from build123d import *

# Parameters (mm, degrees)
SKETCH_1_R       = 11
EXTRUDE_1_DEPTH  = 14
SKETCH_3_R       = 10.95
SKETCH_3_R_2     = 10.9
EXTRUDE_6_DEPTH  = 26
SKETCH_5_R       = 11
SKETCH_5_R_2     = 10.95
SKETCH_5_R_3     = 10.9
EXTRUDE_7_DEPTH  = 11
SKETCH_6_R       = 7
SKETCH_6_R_2     = 6.25
EXTRUDE_8_DEPTH  = 16.5
SKETCH_6_3_R     = 3.75
SKETCH_6_3_R_2   = 3.25
EXTRUDE_9_DEPTH  = 15
FILLET_1_R       = 0.5
FILLET_2_R       = 0.5
SKETCH_8_R       = 9
EXTRUDE_10_DEPTH = 15
SKETCH_9_R       = 4.762822891
EXTRUDE_11_DEPTH = 15
CHAMFER_1_SIZE   = 4
CHAMFER_1_SIZE2  = 2.800830153


with BuildPart() as part:
    # Sketch 1 → Extrude 1 (new body)
    with BuildSketch(Plane(origin=(0, 0, 0), x_dir=(1, 0, 0), z_dir=(0, 1, 0))):
        with Locations(Location((0, 0, 0), (0, 0, 270))):
            Circle(SKETCH_1_R)
    extrude(amount=EXTRUDE_1_DEPTH)

    # Sketch 3 → Extrude 6 (add)
    with BuildSketch(Plane(origin=(0, 14, 0), x_dir=(1, 0, 0), z_dir=(0, 1, 0))):
        with Locations(Location((0, 0, 0), (0, 0, 90))):
            Circle(SKETCH_3_R)
        with Locations(Location((0, 0, 0), (0, 0, 90))):
            Circle(SKETCH_3_R_2, mode=Mode.SUBTRACT)
    extrude(amount=EXTRUDE_6_DEPTH)

    # Sketch 5 → Extrude 7 (add)
    # profile 1 of 3: a face of its own
    with BuildSketch(Plane(origin=(0, 40, 0), x_dir=(1, 0, 0), z_dir=(0, 1, 0))):
        with Locations(Location((0, 0, 0), (0, 0, 270))):
            Circle(SKETCH_5_R)
        with Locations(Location((0, 0, 0), (0, 0, 90))):
            Circle(SKETCH_5_R_2, mode=Mode.SUBTRACT)
    # profile 2 of 3: a face of its own
    with BuildSketch(Plane(origin=(0, 40, 0), x_dir=(1, 0, 0), z_dir=(0, 1, 0))):
        with Locations(Location((0, 0, 0), (0, 0, 90))):
            Circle(SKETCH_5_R_2)
        with Locations(Location((0, 0, 0), (0, 0, 90))):
            Circle(SKETCH_5_R_3, mode=Mode.SUBTRACT)
    # profile 3 of 3: a face of its own
    with BuildSketch(Plane(origin=(0, 40, 0), x_dir=(1, 0, 0), z_dir=(0, 1, 0))):
        with Locations(Location((0, 0, 0), (0, 0, 90))):
            Circle(SKETCH_5_R_3)
    extrude(amount=EXTRUDE_7_DEPTH)

    # Sketch 6 → Extrude 8 (add)
    with BuildSketch(Plane(origin=(0, 51, 0), x_dir=(1, 0, 0), z_dir=(0, 1, 0))):
        with Locations(Location((0, 0, 0), (0, 0, 270))):
            Circle(SKETCH_6_R)
        with Locations(Location((0, 0, 0), (0, 0, 270))):
            Circle(SKETCH_6_R_2, mode=Mode.SUBTRACT)
    extrude(amount=EXTRUDE_8_DEPTH)

    # Sketch 6_3 → Extrude 9 (add)
    with BuildSketch(Plane(origin=(0, 51, 0), x_dir=(1, 0, 0), z_dir=(0, 1, 0))):
        with Locations(Location((0, 0, 0), (0, 0, 270))):
            Circle(SKETCH_6_3_R)
        with Locations(Location((0, 0, 0), (0, 0, 270))):
            Circle(SKETCH_6_3_R_2, mode=Mode.SUBTRACT)
    extrude(amount=EXTRUDE_9_DEPTH)

    # Fillet 1
    fillet_1_edges = [part.edges().sort_by_distance(p)[0] for p in [
        (0, 51, -11),
    ]]
    fillet(fillet_1_edges, radius=FILLET_1_R)

    # Fillet 2
    fillet_2_edges = [part.edges().sort_by_distance(p)[0] for p in [
        (0, 67.5, -7),
    ]]
    fillet(fillet_2_edges, radius=FILLET_2_R)

    # Sketch 8 → Extrude 10 (add)
    with BuildSketch(Plane(origin=(0, 14, 0), x_dir=(1, 0, 0), z_dir=(0, 1, 0))):
        with Locations(Location((0, 0, 0), (0, 0, 270))):
            Circle(SKETCH_8_R)
    extrude(amount=EXTRUDE_10_DEPTH)

    # Sketch 9 → Extrude 11 (add)
    with BuildSketch(Plane(origin=(0, 29, 0), x_dir=(1, 0, 0), z_dir=(0, 1, 0))):
        with Locations(Location((0, 0, 0), (0, 0, 270))):
            Circle(SKETCH_9_R)
    extrude(amount=EXTRUDE_11_DEPTH)

    # Chamfer 1
    chamfer_1_edges = [part.edges().sort_by_distance(p)[0] for p in [
        (0, 29, -4.762822891),
    ]]
    chamfer_1_side = [part.faces().sort_by_distance(p)[0] for p in [
        (0, 29, -8.745441559),
    ]]
    chamfer(chamfer_1_edges, length=CHAMFER_1_SIZE, length2=CHAMFER_1_SIZE2, reference=chamfer_1_side[0])


solid = part.part
Can you work these out from the model? Positions are in its coordinate system, mm. A direction names the side the tool comes from. Give positions to 0.01 mm unless a question says otherwise; leave off trailing zeros. Loops run counter-clockwise (first coordinate to the right, second up) from the corner with the lowest first, then second, coordinate; pieces in that order, holes last. Notation, with made-up numbers: (61.25, 49) -> (104.25, 49) arc R11 ccw to (104.25, 65) -> close; hole circle Ø3 at (88.5, 85). An arc over 180 degrees is marked (long way). Use one line per item in the form item = value.
1) If we section it at B-B (z = 0): Count the separate pieces of the cut face and the enclosed holes in it, plus the area to 3 significant figures.
Answers:
separate_pieces = 1
enclosed_holes = 2
area = 978 mm²
2) Will these pins go through, and if not, where does the flat tip stop? pin 1 (5 mm diameter, centred on x = -6.5, y = 44.5, fed in from -Z); pin 2 (12 mm diameter, centred on x = 2, y = 28.5, fed in from +Z); pin 3 (2 mm diameter, centred on y = 56, z = 1.5, fed in from -X).
Answers:
pin_1 = -10.25
pin_2 = 10.95
pin_3 = -6.98
3) For faces 1 (the face through (9, 14, 2)), 2 (the face through (-10.74, 45.18, -2.38)), 3 (the face through (0, 51, 0)), which set-ups out of +Z, -Z, +X, -X, +Y, -Y let a thin tool reach every point of the face, with its end or its side?
Answers:
face_1 = none
face_2 = +Y, -Y
face_3 = +Y
4) I need wall thicknesses on line 1 along X through (y, z) = (62.75, 0); line 2 along Z through (x, y) = (-1, 53); line 3 along Y through (x, z) = (-9.5, 1.75). Which ranges of each line are inside material? Lowest first, please.
Answers:
line_1 = -7 to -6.25, -3.75 to -3.25, 3.25 to 3.75, 6.25 to 7
line_2 = -6.93 to -6.17, -3.61 to -3.09, 3.09 to 3.61, 6.17 to 6.93
line_3 = 0 to 14, 40 to 51
5) If we section it at A-A (y = 33): Please give me the cut outline in (x, z), plus the area to 3 significant figures.
Answers:
outline = circle Ø21.9 at (0, 0); circle Ø9.53 at (0, 0); hole circle Ø21.8 at (0, 0)
area = 74.7 mm²
6) If we section it at D-D (y = 47): Please give me the cut outline in (x, z), plus the area to 3 significant figures.
Answers:
outline = circle Ø22 at (0, 0)
area = 380 mm²
7) We'd pull the mould along X, two halves only. Please class faces 4 (the face through (0, 0, 0)), 5 (the face through (-6.834, 58.888, -1.517)), 6 (the face through (-1.978, 58.395, -2.579)): released by +X, released by -X, zero draft, split by the parting line, or undercut.
Answers:
face_4 = zero draft
face_5 = split by the parting line
face_6 = undercut
